Design review of the part shown in the three views and the two pictorial views. Dimensions are in mm from the part's minimum x, y and z. A direction names the side the tool comes from. Coordinates: 2 decimals unless noted, no trailing zeros. Order: outer loops, then holes, each group sorted by start corner. A loop starts at its lowest first (then second) coordinate and runs counter-clockwise, first axis right, second up. Notation, with made-up numbers: (25, 21) -> (32, 21) arc R16 cw to (32, 34) -> close; hole circle Ø1 at (-9, 84). An arc over 180 degrees is marked (long way). Answer as a JSON object with one key per item and string values. Group by question number.
1) Add section D-D, the plane y = 8.25. Write out the cut boundary in (x, z).
2) Draft analysis for pull direction Z (two halves, no side actions). For the marked faces 3, 4 and 5, state which applies: +Z half, -Z half, draft (parallel to the pull), parting line (faces both ways), or undercut.
3) Wall thickness on L1, parallel to Z at x = 4, y = 2; L2, parallel to X at y = 2.25, z = 4; L3, parallel to X at y = 6.75, z = 5.5: over which ranges is each line inside the solid? List them lowest first.
4) Add section C-C, the plane z = 14. Write out the cut boundary in (x, y).
5) Add section A-A, the plane y = 2.5. Write out the cut boundary in (x, z).
6) Add section B-B, the plane x = 4. Write out the cut boundary in (y, z), then the cut area to 3 significant figures.
7) For pin 1 (1 mm diameter, centred on x = 13.5, y = 6.5, fed in from -Z); pin 2 (2 mm diameter, centred on x = 8.5, z = 5, fed in from -Y); pin 3 (3 mm diameter, centred on x = 4, z = 14, fed in from +Y), all flat-tipped, find the tip position at first contact; note any pin that passes through.
8) Machinability: for the marked faces 1 and 2, which of the approach directions +Z, -Z, +X, -X, +Y, -Y give a long, thin tool a straight path to every point of the face, cutting with its end or side? Answer none if there is none.
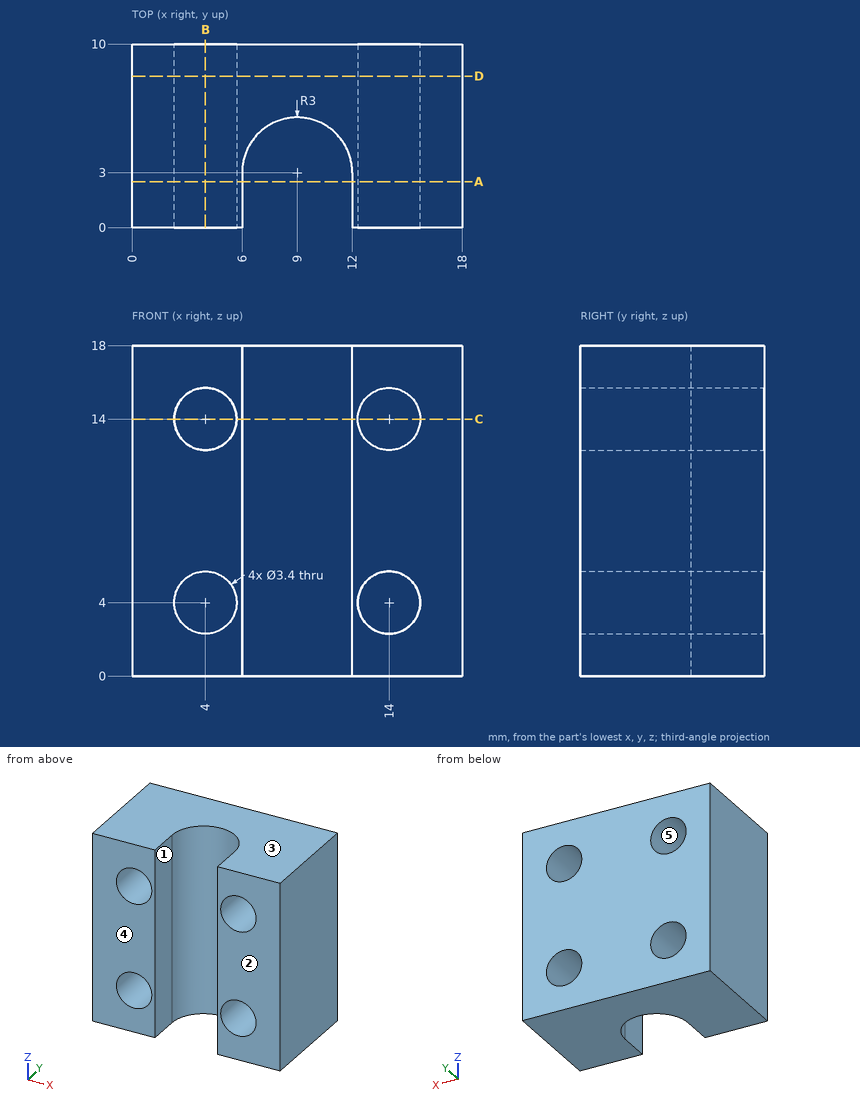
Output values:
{
 "1": {"outline": "(0, 0) -> (18, 0) -> (18, 18) -> (0, 18) -> close; hole circle Ø3.4 at (4, 4); hole circle Ø3.4 at (4, 14); hole circle Ø3.4 at (14, 4); hole circle Ø3.4 at (14, 14)"},
 "2": {"face 3": "+Z half", "face 4": "draft", "face 5": "undercut"},
 "3": {"L1": "z = 0 to 2.3, 5.7 to 12.3, 15.7 to 18", "L2": "x = 0 to 2.3, 5.7 to 6, 12 to 12.3, 15.7 to 18", "L3": "x = 0 to 3.2, 4.8 to 13.2, 14.8 to 18"},
 "4": {"outline": "(0, 0) -> (2.3, 0) -> (2.3, 10) -> (0, 10) -> close; (5.7, 0) -> (6, 0) -> (6, 3) arc R3 cw to (12, 3) -> (12, 0) -> (12.3, 0) -> (12.3, 10) -> (5.7, 10) -> close; (15.7, 0) -> (18, 0) -> (18, 10) -> (15.7, 10) -> close"},
 "5": {"outline": "(0, 0) -> (6, 0) -> (6, 18) -> (0, 18) -> close; (12, 0) -> (18, 0) -> (18, 18) -> (12, 18) -> close; hole circle Ø3.4 at (4, 4); hole circle Ø3.4 at (4, 14); hole circle Ø3.4 at (14, 4); hole circle Ø3.4 at (14, 14)"},
 "6": {"outline": "(0, 0) -> (10, 0) -> (10, 2.3) -> (0, 2.3) -> close; (0, 5.7) -> (10, 5.7) -> (10, 12.3) -> (0, 12.3) -> close; (0, 15.7) -> (10, 15.7) -> (10, 18) -> (0, 18) -> close", "area": "112 mm²"},
 "7": {"pin 1": "stops at z = 0", "pin 2": "stops at y = 5.6", "pin 3": "passes through"},
 "8": {"face 1": "+Z, -Z, -Y", "face 2": "+Z, -Z, +X, -X, -Y"}
}
